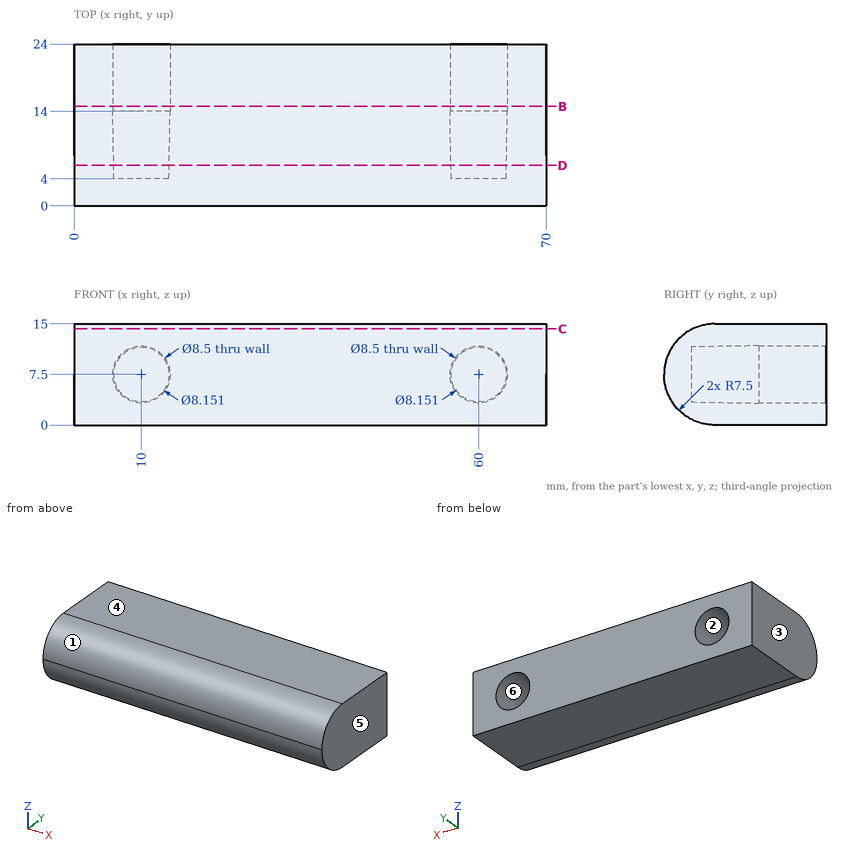
The drawing under review shows one solid part. Ordinate dimensions are in mm from its lowest x, y, z. A direction names the side the tool comes from. Coordinates: 2 decimals unless noted, no trailing zeros. Order: outer loops, then holes, each group sorted by start corner. A loop starts at its lowest first (then second) coordinate and runs counter-clockwise, first axis right, second up. Notation, with made-up numbers: (-20.5, 11.25) -> (-9.5, 11.25) arc R18 ccw to (-9.5, 45.25) -> close; hole circle Ø6 at (-7.5, 48.5). An arc over 180 degrees is marked (long way). Use CSV: the item, a comma, the result in double quotes. Start each with the question number.
Item 1: We need section C-C, the plane z = 14.25. Give the boundary of the cut face in (x, y), then the cut area to 3 significant figures.
Item 2: Draft analysis for pull direction X (two halves, no side actions). For the marked faces 3, 4, 5 and 6, state which applies: pulls with the +X half, pulls with the -X half, needs draft (parallel to the pull), parting line crosses it, or undercut.
Item 3: We need section D-D, the plane y = 6. Give the boundary of the cut face in (x, z), then the cut area to 3 significant figures.
Item 4: For the marked faces 1 and 2, list the 3-axis set-ups (+Z, -Z, +X, -X, +Y, -Y) from which the entire face can be reached by the end or side of a thin tool; tool diameter is ignored.
Item 5: We need section B-B, the plane y = 14.75. Give the boundary of the cut face in (x, z).
Item 6: Insertion check: pin 1 (4 mm diameter, centred on x = 59.5, z = 6.5, fed in from +Y). The pin has a flat end and moves straight along its axis. Give the tip position at first contact, or say it passes through.
Item 7: Wall thickness on probe 1 along X at (y, z) = (17.25, 7.5); probe 2 along X at (y, z) = (16.75, 10.25); probe 3 along Y at (x, z) = (30.5, 7.25): over which ranges is each line inside the solid? List them lowest first.
Derived:
1,outline,"(0, 4.23) -> (70, 4.23) -> (70, 24) -> (0, 24) -> close"
1,area,"1,380 mm^2"
2,face 3,"pulls with the -X half"
2,face 4,"needs draft"
2,face 5,"pulls with the +X half"
2,face 6,"undercut"
3,outline,"(0, 0.15) -> (70, 0.15) -> (70, 14.85) -> (0, 14.85) -> close; hole circle Ø8.22 at (10, 7.5); hole circle Ø8.22 at (60, 7.5)"
3,area,"923 mm^2"
4,face 1,"+Z, +X, -X, -Y"
4,face 2,"+Y"
5,outline,"(0, 0) -> (70, 0) -> (70, 15) -> (0, 15) -> close; hole circle Ø8.5 at (10, 7.5); hole circle Ø8.5 at (60, 7.5)"
6,pin 1,"stops at y = 4"
7,probe 1,"x = 0 to 5.75, 14.25 to 55.75, 64.25 to 70"
7,probe 2,"x = 0 to 6.76, 13.24 to 56.76, 63.24 to 70"
7,probe 3,"y = 0 to 24"
